from build123d import *

# Parameters (mm, degrees)
SKETCH1_W           = 67.31
SKETCH1_H           = 146.05
BOSS_EXTRUDE1_DEPTH = 5.9944
SKETCH2_W           = 6.604
SKETCH2_H           = 4.445
CUT_EXTRUDE1_DEPTH  = 6.9944
SKETCH3_W           = 25.4
SKETCH3_H           = 22.225
SKETCH3_R           = 6.35
BOSS_EXTRUDE2_DEPTH = 5.9944


with BuildPart() as part:
    # Sketch1 → Boss-Extrude1 (new body)
    with BuildSketch(Plane.XY):
        Polygon((0, 19.05), (0, 177.8), (6.35, 177.8), (73.66, 177.8), (80.01, 177.8), (80.01, 19.05), (60.96, 19.05), (60.96, 0), (19.05, 0), (19.05, 19.05), align=None)
        with Locations((40.005, 98.425)):
            Rectangle(SKETCH1_W, SKETCH1_H, mode=Mode.SUBTRACT)
    extrude(amount=-BOSS_EXTRUDE1_DEPTH)

    # Sketch2 → Cut-Extrude1 (cut, through all)
    with BuildSketch(Plane.XY):
        with Locations((6.35, 33.9725)):
            Rectangle(SKETCH2_W, SKETCH2_H)
        with Locations((6.35, 47.3075)):
            Rectangle(SKETCH2_W, SKETCH2_H)
        with Locations((6.35, 60.6425)):
            Rectangle(SKETCH2_W, SKETCH2_H)
        with Locations((6.35, 73.9775)):
            Rectangle(SKETCH2_W, SKETCH2_H)
        with Locations((6.35, 87.3125)):
            Rectangle(SKETCH2_W, SKETCH2_H)
        with Locations((6.35, 100.6475)):
            Rectangle(SKETCH2_W, SKETCH2_H)
        with Locations((6.35, 113.9825)):
            Rectangle(SKETCH2_W, SKETCH2_H)
        with Locations((6.35, 127.3175)):
            Rectangle(SKETCH2_W, SKETCH2_H)
        with Locations((6.35, 140.6525)):
            Rectangle(SKETCH2_W, SKETCH2_H)
        with Locations((6.35, 153.9875)):
            Rectangle(SKETCH2_W, SKETCH2_H)
        with Locations((73.66, 153.9875)):
            Rectangle(SKETCH2_W, SKETCH2_H)
        with Locations((73.66, 140.6525)):
            Rectangle(SKETCH2_W, SKETCH2_H)
        with Locations((73.66, 127.3175)):
            Rectangle(SKETCH2_W, SKETCH2_H)
        with Locations((73.66, 113.9825)):
            Rectangle(SKETCH2_W, SKETCH2_H)
        with Locations((73.66, 100.6475)):
            Rectangle(SKETCH2_W, SKETCH2_H)
        with Locations((73.66, 87.3125)):
            Rectangle(SKETCH2_W, SKETCH2_H)
        with Locations((73.66, 73.9775)):
            Rectangle(SKETCH2_W, SKETCH2_H)
        with Locations((73.66, 60.6425)):
            Rectangle(SKETCH2_W, SKETCH2_H)
        with Locations((73.66, 47.3075)):
            Rectangle(SKETCH2_W, SKETCH2_H)
        with Locations((73.66, 33.9725)):
            Rectangle(SKETCH2_W, SKETCH2_H)
    extrude(amount=-CUT_EXTRUDE1_DEPTH, mode=Mode.SUBTRACT)

    # Sketch3 → Boss-Extrude2 (add)
    with BuildSketch(Plane.XY):
        with Locations((40.005, 188.9125)):
            Rectangle(SKETCH3_W, SKETCH3_H)
        with Locations((40.005, 188.9125)):
            Circle(SKETCH3_R, mode=Mode.SUBTRACT)
    extrude(amount=-BOSS_EXTRUDE2_DEPTH)


solid = part.part
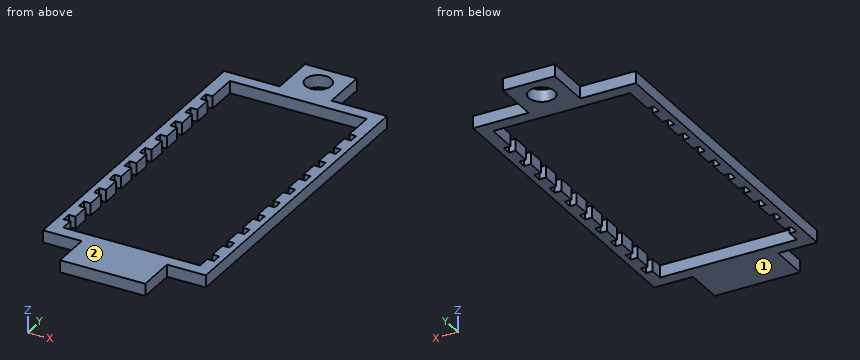
Design review of the part built by this model. Coordinates are the model's own, in mm. Face numbers are marked on the shaded views. Give positions to 0.01 mm unless a question says otherwise; leave off trailing zeros. Loops run counter-clockwise (first coordinate to the right, second up) from the corner with the lowest first, then second, coordinate; pieces in that order, holes last. Notation, with made-up numbers: (23.5, 40) - (68.5, 40) arc R30 ccw to (68.5, 66) - close; hole circle Ø5 at (62.25, 56). An arc over 180 degrees is marked (long way). Use CSV: the item, a comma, the result in double quotes. Start each with the question number.
1. Wall thickness on L1, parallel to X at y = 129, z = -4.25; L2, parallel to Y at x = 62.5, z = -4.55; L3, parallel to Y at x = 25, z = -2.5: over which ranges is each line inside the solid? List them lowest first.
2. Insertion check: P1, Ø1.8, axis at x = 15.5, z = -4, coming from the +Y side; P2, Ø3.5, axis at x = 76, z = -2.5, coming from the -Y side. Each pin has a flat end and moves straight along its axis. Give the tip position at first contact, or say it passes through.
3. Add section D-D (z = -3.95). Count the separate pieces of the cut face and the enclosed holes in it, plus the area to 3 significant figures.
4. Add section B-B (y = 141). State the section outline as (x, z) points.
5. Add section C-C (x = 44.5). State the section outline as (y, z) points (3 decimals).
6. Add section A-A (x = 58). State the section outline as (y, z) points, plus the area to 3 significant figures.
7. Draft analysis for pull direction Z (two halves, no side actions). For the marked faces 1 and 2, state which applies: released by +Z, released by -Z, zero draft, split by the parting line, or undercut.
Results found:
1,L1,"x = 0 to 3.05, 76.96 to 80.01"
1,L2,"y = 19.05 to 25.4, 171.45 to 177.8"
1,L3,"y = 0 to 25.4, 171.45 to 177.8"
2,P1,"stops at y = 177.8"
2,P2,"stops at y = 19.05"
3,separate pieces,"1"
3,enclosed holes,"2"
3,area,"3,810 mm²"
4,outline,"(0, -5.99) - (3.05, -5.99) - (3.05, 0) - (0, 0) - close; (76.96, -5.99) - (80.01, -5.99) - (80.01, 0) - (76.96, 0) - close"
5,outline,"(0, -5.994) - (25.4, -5.994) - (25.4, 0) - (0, 0) - close; (171.45, -5.994) - (184.427, -5.994) - (184.427, 0) - (171.45, 0) - close; (193.398, -5.994) - (200.025, -5.994) - (200.025, 0) - (193.398, 0) - close"
6,outline,"(0, -5.99) - (25.4, -5.99) - (25.4, 0) - (0, 0) - close; (171.45, -5.99) - (177.8, -5.99) - (177.8, 0) - (171.45, 0) - close"
6,area,"190 mm²"
7,face 1,"released by -Z"
7,face 2,"released by +Z"
